```python
from build123d import *

# Parameters (mm, degrees)
SKETCH_1_W               = 60
SKETCH_1_H               = 60
EXTRUDE_2_DEPTH          = 30
FILLET_4_R               = 10
FILLET_5_R               = 10
SKETCH_5_W               = 47
SKETCH_5_H               = 47
CUT_EXTRUDE_4_DEPTH      = 47
CHAMFER_3_SIZE           = 15
CHAMFER_4_SIZE           = 15
CUT_EXTRUDE_START        = -4
SKETCH_6_R               = 40
CUT_EXTRUDE_5_DEPTH      = 5
SKETCH_7_R               = 10
SKETCH_7_W               = 5
SKETCH_7_H               = 4
CUT_EXTRUDE_6_DEPTH      = 13
PATTERN_CIRCULAR_5_COUNT = 3


with BuildPart() as part:
    # 草图1 → 凸台-拉伸2 (new, symmetric)
    with BuildSketch(Plane(origin=(0, 0, 0), x_dir=(1, 0, 0), z_dir=(0, 1, 0))):
        Rectangle(SKETCH_1_W, SKETCH_1_H)
    extrude(amount=EXTRUDE_2_DEPTH, both=True)

    # 圆角4
    fillet_4_edges = [part.edges().sort_by_distance(p)[0] for p in [
        (0, -30, 30),
        (-30, -30, 0),
    ]]
    fillet(fillet_4_edges, radius=FILLET_4_R)

    # 圆角5
    # the kernel refuses this fillet: 10 mm, written as the material it takes off along each edge
    with BuildSketch(Plane(origin=(-30, -45, 30), x_dir=(0, 0, -1), z_dir=(0, 1, 0))) as fillet_5_piece_1:
        with BuildLine():
            CenterArc((FILLET_5_R, -FILLET_5_R), FILLET_5_R, 90, 90)
            Line((0, -FILLET_5_R), (0, 0))
            Line((0, 0), (FILLET_5_R, 0))
        make_face()
    extrude(amount=100, mode=Mode.SUBTRACT)

    # 草图5 → 切除-拉伸4 (cut)
    with BuildSketch(Plane(origin=(0, 30, 0), x_dir=(1, 0, 0), z_dir=(0, 1, 0))):
        with Locations((6.5, 6.5)):
            Rectangle(SKETCH_5_W, SKETCH_5_H)
    extrude(amount=-CUT_EXTRUDE_4_DEPTH, mode=Mode.SUBTRACT)

    # 倒角3
    chamfer_3_edges = [part.edges().sort_by_distance(p)[0] for p in [
        (6.5, -17, 17),
        (-17, -17, -6.5),
    ]]
    chamfer(chamfer_3_edges, length=CHAMFER_3_SIZE)

    # 倒角4
    chamfer_4_edges = [part.edges().sort_by_distance(p)[0] for p in [
        (-17, 14, 17),
    ]]
    chamfer(chamfer_4_edges, length=CHAMFER_4_SIZE)

    # 草图6 → 切除-拉伸5 (cut)
    with BuildSketch(Plane.XY.offset(30).offset(CUT_EXTRUDE_START)):
        with Locations((30, 30)):
            Circle(SKETCH_6_R)
    cut_extrude_5 = extrude(amount=-CUT_EXTRUDE_5_DEPTH, mode=Mode.SUBTRACT)

    # 草图7 → 切除-拉伸6 (cut)
    with BuildSketch(Plane.XY.offset(30)):
        with Locations((17, 30)):
            Circle(SKETCH_7_R)
        with Locations((27.5, 8)):
            Rectangle(SKETCH_7_W, SKETCH_7_H)
    cut_extrude_6 = extrude(amount=-CUT_EXTRUDE_6_DEPTH, mode=Mode.SUBTRACT)

    # 阵列(圆周)5: 切除-拉伸5, 切除-拉伸6 ×3 about axis
    pattern_circular_5_axis = Axis((0, 0, 0), (-0.5773502691896262, -0.5773502691896245, 0.5773502691896266))
    add([cut_extrude_5.rotate(pattern_circular_5_axis, i * 360 / PATTERN_CIRCULAR_5_COUNT) for i in range(1, PATTERN_CIRCULAR_5_COUNT)], mode=Mode.SUBTRACT)
    add([cut_extrude_6.rotate(pattern_circular_5_axis, i * 360 / PATTERN_CIRCULAR_5_COUNT) for i in range(1, PATTERN_CIRCULAR_5_COUNT)], mode=Mode.SUBTRACT)


solid = part.part
```
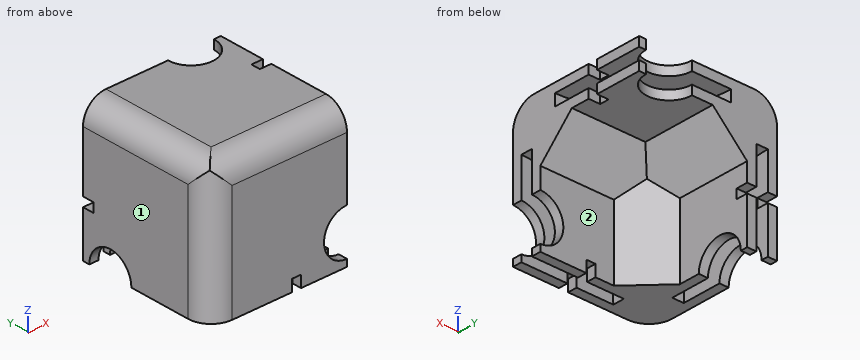
The model under review builds one solid part; all positions refer to its coordinate system, in mm. Face numbers are marked on the shaded views. A direction names the side the tool comes from. Coordinates: 2 decimals unless noted, no trailing zeros. Write each loop counter-clockwise with the first axis right and the second up, starting at its lowest first coordinate (ties: lowest second). Pieces come first, ordered by that corner, then holes.
1) Machinability: for the marked faces 1 and 2, which of the approach directions +Z, -Z, +X, -X, +Y, -Y give a long, thin tool a straight path to every point of the face, cutting with its end or side? Answer none if there is none.
2) We need section A-A on y = -15. State the section outline as (x, z) points.
3) We need section C-C on x = 8.5. State the section outline as (y, z) points, then the cut area to 3 significant figures.
4) Clearance check with flat-ended pins moving along their axes: pin 1 Ø6 at (x, y) = (7.5, -19.5) entering from -Z; pin 2 Ø8 at (x, y) = (19, 22.5) entering from -Z; pin 3 Ø2 at (x, y) = (-28.5, 26.5) entering from +Z; pin 4 Ø20 at (y, z) = (4.5, -6.5) entering from +X. State where each tip first meets the part, or that it passes through.
5) We need section B-B on z = 12.5. State the section outline as (x, y) points.
6) To check wall thickness, follow probe 1 along Y at (x, z) = (-0.5, -12); probe 2 along Y at (x, z) = (13, 9). State the ranges of each line that lie inside material, in increasing order.
7) We need section D-D on y = 1. State the section outline as (x, z) points, then the cut area to 3 significant figures.
Answer list:
1. face 1: +Z, -Z, -X, +Y, -Y
1. face 2: -Z, +X, +Y
2. outline: (-30, -30) - (-4, -30) - (-4, 4) - (30, 4) - (30, 30) - (-20, 30) arc R10 ccw to (-30, 20) - close
3. outline: (-30, -25) - (-26, -25) - (-26, 3.73) - (-21, 3.73) - (-21, -25) - (-17, -25) - (-17, 2) - (-2, 17) - (24.73, 17) - (24.73, 21) - (-3.73, 21) - (-3.73, 26) - (24.73, 26) - (24.73, 30) - (-20, 30) arc R10 ccw to (-30, 20) - close
3. area: 1,060 mm2
4. pin 1: stops at z = -30
4. pin 2: stops at z = 17
4. pin 3: stops at z = 26.61
4. pin 4: stops at x = -13.5
5. outline: (-30, -20) arc R10 ccw to (-20, -30) - (30, -30) - (30, -6.5) - (-6.5, -6.5) - (-6.5, 30) - (-30, 30) - close
6. probe 1: y = -30 to -26, -21 to -17
6. probe 2: y = -30 to -10
7. outline: (-30, -30) - (-26, -30) - (-26, -2.45) - (-21, -2.45) - (-21, -30) - (-17, -30) - (-17, 2) - (-2, 17) - (30, 17) - (30, 21) - (2.45, 21) - (2.45, 26) - (30, 26) - (30, 30) - (-20, 30) arc R10 ccw to (-30, 20) - close
7. area: 1,210 mm2
